```python
from build123d import *

# Parameters (mm, degrees)
F1_R      = 26.2655065646
F2_DEPTH  = 25.4
F3_DEPTH  = 25.4
F4_DEPTH  = 25.4
F5_R      = 27.8330469694
F6_DEPTH  = 22.352
F8_W      = 33.9538175613
F8_H      = 12.0044872165
F9_DEPTH  = 7.112
F11_R     = 3.0284549087
F13_DEPTH = 1.016
F14_R     = 8.9450781304
F14_R_2   = 3.0284549087
F15_DEPTH = 0.762
F16_R     = 25.222843128
F17_DEPTH = 0.762
F19_R     = 3.7698908718
F20_DEPTH = 2.286
F21_W     = 32.6801389456
F21_H     = 11.2690133974
F22_DEPTH = 0.762
F24_DEPTH = 64.008
F25_DEPTH = 12.954
F10_W     = 77.0918577909
F10_H     = 47.0512080938
F26_DEPTH = 1.016
F27_W     = 15.3993144631
F27_H     = 17.6025833935
F27_W_2   = 9.2281326652
F27_H_2   = 11.5900784731
F28_DEPTH = 2.54


with BuildPart() as f2:
    # F1 (on face) → F2 (new body)
    with BuildSketch(Plane.XZ):
        with Locations((-2.629437251, -9.2030279338)):
            Circle(F1_R)
    extrude(amount=F2_DEPTH)

    # F0 (on Front) → F3 (join)
    with BuildSketch(Plane.XZ):
        Polygon((-50.7105626166, 23.4771128744), (-60.85267663, 23.4771128744), (-60.85267663, -40.5684486032), (63.2942989469, -40.5684486032), (63.2942989469, 23.4771128744), (-24.228380993, 23.4771128744), align=None)
    extrude(amount=-F3_DEPTH)

    # F4 (add): a face of the model
    f4_faces = [f2.faces().sort_by_distance(p)[0] for p in [
        (1.2208111584, 0, 22.0801767452),
    ]]
    extrude(f4_faces, amount=F4_DEPTH)

    # F5 (on face) → F6 (join)
    with BuildSketch(Plane.XZ.offset(25.4)):
        with Locations((0, -9.5786619931)):
            Circle(F5_R)
    extrude(amount=F6_DEPTH)

    # F8 (on face) → F9 (join)
    with BuildSketch(Plane.XY.offset(23.4771128744)):
        with Locations((-39.6948745474, -10.6415767223)):
            Rectangle(F8_W, F8_H)
    extrude(amount=F9_DEPTH)

    # F11 (on face) → F13 (join)
    with BuildSketch(Plane(origin=(0, 25.4, 0), x_dir=(-1, 0, 0), z_dir=(0, 1, 0))):
        with Locations((41.3197204471, -14.4619019702)):
            Circle(F11_R)
    extrude(amount=F13_DEPTH)

    # F14 (on face) → F15 (join)
    with BuildSketch(Plane(origin=(0, 25.4, 0), x_dir=(-1, 0, 0), z_dir=(0, 1, 0))):
        with Locations((41.3197204471, -14.4619019702)):
            Circle(F14_R)
        with Locations((41.3197204471, -14.4619019702)):
            Circle(F14_R_2, mode=Mode.SUBTRACT)
    extrude(amount=-F15_DEPTH)

    # F16 (on face) → F17 (join)
    with BuildSketch(Plane.XZ.offset(47.752)):
        with Locations((0, -9.5786619931)):
            Circle(F16_R)
    extrude(amount=F17_DEPTH)

    # F19 (on face) → F20 (join)
    with BuildSketch(Plane.XY.offset(23.4771128744)):
        with Locations((54.2063601315, -28.089210391)):
            Circle(F19_R)
    extrude(amount=F20_DEPTH)

    # F21 (on face) → F22 (join)
    with BuildSketch(Plane.XZ.offset(25.4)):
        with Locations((-42.822252959, 15.4009857215)):
            Rectangle(F21_W, F21_H)
    extrude(amount=F22_DEPTH)

    # F23 (on face) → F24 (join)
    with BuildSketch(Plane.XY.offset(23.4771128744)):
        with BuildLine():
            ThreePointArc((46.1644789676, -25.4), (53.7686719478, -36.0181838323), (63.4942040761, -27.3013263941))
            ThreePointArc((63.4942040761, -27.3013263941), (63.4418971886, -26.3449585915), (63.2856005331, -25.4))
            Line((63.2856005331, -25.4), (46.1644789676, -25.4))
        make_face()
        with BuildLine():
            Line((46.1644789676, -25.4), (63.2856005331, -25.4))
            ThreePointArc((63.2856005331, -25.4), (54.7250397503, -18.5321620683), (46.1644789676, -25.4))
        make_face()
    extrude(amount=-F24_DEPTH)

    # F25 (add): a face of the model
    f25_faces = [f2.faces().sort_by_distance(p)[0] for p in [
        (0, -48.514, -9.5786619931),
    ]]
    extrude(f25_faces, amount=F25_DEPTH)

    # F10 (on face) → F26 (join)
    with BuildSketch(Plane(origin=(0, 25.4, 0), x_dir=(-1, 0, 0), z_dir=(0, 1, 0))):
        with Locations((-17.513666302, -9.6154874191)):
            Rectangle(F10_W, F10_H)
    extrude(amount=F26_DEPTH)

    # F27 (on face) → F28 (join)
    with BuildSketch(Plane(origin=(0, 25.4, 0), x_dir=(-1, 0, 0), z_dir=(0, 1, 0))):
        with Locations((41.0268343985, 12.4612255022)):
            Rectangle(F27_W, F27_H)
        with Locations((41.0268343985, 12.4612255022)):
            Rectangle(F27_W_2, F27_H_2, mode=Mode.SUBTRACT)
    extrude(amount=F28_DEPTH)


solid = f2.part
```
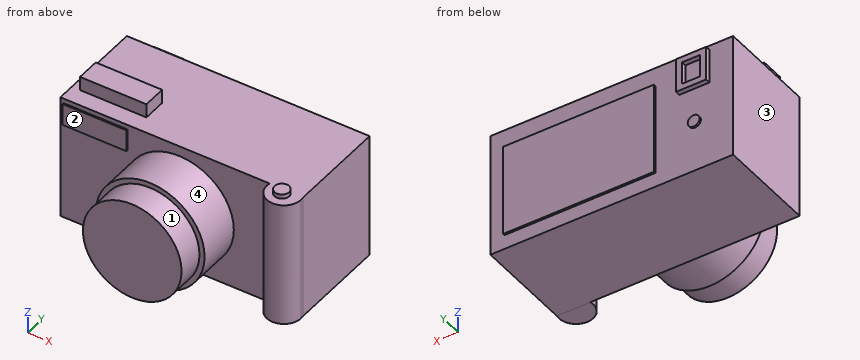
For this review, take the finished solid that the model builds, in its own axes (mm). Face numbers are marked on the shaded views. Coordinates: 2 decimals unless noted, no trailing zeros. Loops run counter-clockwise (first coordinate to the right, second up) from the corner with the lowest first, then second, coordinate; pieces in that order, holes last.
1. For line 1 (Z direction, x = 17, y = 17.5); line 2 (X direction, y = 2.5, z = -35); line 3 (Y direction, x = -1, z = -9), list the stretches that pass through material, from the lowest coordinate up.
2. Add section C-C, the plane y = 7. Give the boundary of the cut face in (x, z).
3. Mouldability with a two-part tool opening along X and no side actions: class the marked faces 1, 2, 3 and 4 as +X half, -X half, draft (parallel to the pull), parting line (faces both ways), or undercut.
4. Insertion check: P1, Ø0.8, axis at x = -43, y = 27, coming from the +Z side; P2, Ø6.5, axis at x = -41.5, z = -13.5, coming from the +Y side; P3, Ø6, axis at x = 18.5, y = -51, coming from the +Z side. Each pin has a flat end and moves straight along its axis. Give the tip position at first contact, or say it passes through.
5. Add section D-D, the plane x = -14. Give the boundary of the cut face in (y, z), then the cut area to 3 significant figures.
6. Add section A-A, the plane x = 34.5. Give the boundary of the cut face in (y, z).
Result:
1. line 1: z = -40.57 to 23.48
1. line 2: x = -60.85 to 63.29
1. line 3: y = -61.47 to 26.42
2. outline: (-60.85, -40.57) - (63.29, -40.57) - (63.29, 23.48) - (-60.85, 23.48) - close
3. face 1: parting line
3. face 2: draft
3. face 3: -X half
3. face 4: undercut
4. P1: stops at z = 21.26
4. P2: stops at y = 26.42
4. P3: stops at z = 10.32
5. outline: (-61.47, -30.56) - (-47.75, -30.56) - (-47.75, -33.63) - (-25.4, -33.63) - (-25.4, -40.57) - (25.4, -40.57) - (25.4, -33.14) - (26.42, -33.14) - (26.42, 13.91) - (25.4, 13.91) - (25.4, 23.48) - (-25.4, 23.48) - (-25.4, 14.48) - (-47.75, 14.48) - (-47.75, 11.4) - (-61.47, 11.4) - close
5. area: 4,950 mm2
6. outline: (-25.4, -40.57) - (25.4, -40.57) - (25.4, -33.14) - (26.42, -33.14) - (26.42, 13.91) - (25.4, 13.91) - (25.4, 23.48) - (-25.4, 23.48) - close
